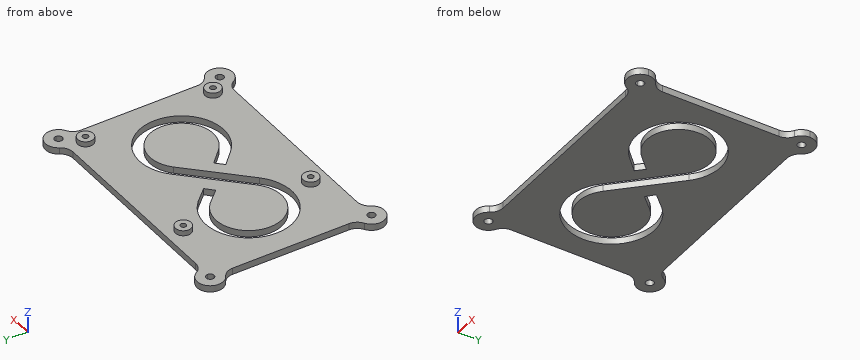
```python
from build123d import *

# Parameters (mm, degrees)
F1_DEPTH = 2.5
F2_R     = 5
F3_R     = 3
F4_DEPTH = 2
F6_D     = 2.2
F6_DEPTH = 3.5
F6_TIP   = 0.6609466809


with BuildPart() as f1:
    # F0 (on Top) → F1 (new body)
    with BuildSketch(Plane.XY):
        with BuildLine():
            ThreePointArc((-45, -26), (-48.5355339059, -34.5355339059), (-40, -31))
            Line((-40, -31), (-43.5, -31))
            ThreePointArc((-43.5, -31), (-46.0606601718, -32.0606601718), (-45, -29.5))
            Line((-45, -29.5), (-45, -26))
        make_face()
        with BuildLine():
            ThreePointArc((-45, -26), (-41.4644660941, -27.4644660941), (-40, -31))
            Line((-40, -31), (40, -31))
            ThreePointArc((40, -31), (41.4644660941, -27.4644660941), (45, -26))
            Line((45, -26), (45, 26))
            ThreePointArc((45, 26), (41.4644660941, 27.4644660941), (40, 31))
            Line((40, 31), (-40, 31))
            ThreePointArc((-40, 31), (-41.4644660941, 27.4644660941), (-45, 26))
            Line((-45, 26), (-45, -26))
        make_face()
        with BuildLine():
            Line((-11.0606601718, -8.9393398282), (8.9393398282, 11.0606601718))
            ThreePointArc((8.9393398282, 11.0606601718), (36.4956890143, -0.3535533906), (8.9393398282, -11.767766953))
            Line((8.9393398282, -11.767766953), (3.7625631329, -6.5909902577))
            Line((3.7625631329, -6.5909902577), (5.1767766953, -5.1767766953))
            Line((5.1767766953, -5.1767766953), (6.5909902577, -3.7625631329))
            Line((6.5909902577, -3.7625631329), (11.767766953, -8.9393398282))
            ThreePointArc((11.767766953, -8.9393398282), (32.4956890143, -0.3535533906), (11.767766953, 8.232233047))
            Line((11.767766953, 8.232233047), (-8.232233047, -11.767766953))
            ThreePointArc((-8.232233047, -11.767766953), (-36.6421356237, 0), (-8.232233047, 11.767766953))
            ThreePointArc((-8.232233047, 11.767766953), (-8.2074655375, 11.7425578811), (-8.1831473235, 11.716915118))
            Line((-8.1831473235, 11.716915118), (-3.3599240188, 6.5401384227))
            Line((-3.3599240188, 6.5401384227), (-4.8232233047, 5.1767766953))
            Line((-4.8232233047, 5.1767766953), (-6.2865225906, 3.8134149679))
            Line((-6.2865225906, 3.8134149679), (-11.0847678218, 8.9633826393))
            ThreePointArc((-11.0847678218, 8.9633826393), (-32.6421241617, -0.0170237742), (-11.0606601718, -8.9393398282))
        make_face(mode=Mode.SUBTRACT)
        with BuildLine():
            Line((-43.5, -31), (-40, -31))
            ThreePointArc((-40, -31), (-41.4644660941, -27.4644660941), (-45, -26))
            Line((-45, -26), (-45, -29.5))
            ThreePointArc((-45, -29.5), (-43.9393398282, -29.9393398282), (-43.5, -31))
        make_face()
        with BuildLine():
            ThreePointArc((45, -26), (41.4644660941, -27.4644660941), (40, -31))
            Line((40, -31), (43.5, -31))
            ThreePointArc((43.5, -31), (43.9393398282, -29.9393398282), (45, -29.5))
            Line((45, -29.5), (45, -26))
        make_face()
        with BuildLine():
            Line((43.5, -31), (40, -31))
            ThreePointArc((40, -31), (45, -36), (50, -31))
            ThreePointArc((50, -31), (48.5355339059, -27.4644660941), (45, -26))
            Line((45, -26), (45, -29.5))
            ThreePointArc((45, -29.5), (46.0606601718, -29.9393398282), (46.5, -31))
            ThreePointArc((46.5, -31), (45, -32.5), (43.5, -31))
        make_face()
        with BuildLine():
            ThreePointArc((-40, 31), (-48.5355339059, 34.5355339059), (-45, 26))
            Line((-45, 26), (-45, 29.5))
            ThreePointArc((-45, 29.5), (-46.0606601718, 32.0606601718), (-43.5, 31))
            Line((-43.5, 31), (-40, 31))
        make_face()
        with BuildLine():
            Line((-45, 29.5), (-45, 26))
            ThreePointArc((-45, 26), (-41.4644660941, 27.4644660941), (-40, 31))
            Line((-40, 31), (-43.5, 31))
            ThreePointArc((-43.5, 31), (-43.9393398282, 29.9393398282), (-45, 29.5))
        make_face()
        with BuildLine():
            ThreePointArc((40, 31), (41.4644660941, 27.4644660941), (45, 26))
            Line((45, 26), (45, 29.5))
            ThreePointArc((45, 29.5), (43.9393398282, 29.9393398282), (43.5, 31))
            Line((43.5, 31), (40, 31))
        make_face()
        with BuildLine():
            Line((45, 29.5), (45, 26))
            ThreePointArc((45, 26), (48.5355339059, 27.4644660941), (50, 31))
            ThreePointArc((50, 31), (45, 36), (40, 31))
            Line((40, 31), (43.5, 31))
            ThreePointArc((43.5, 31), (45, 32.5), (46.5, 31))
            ThreePointArc((46.5, 31), (46.0606601718, 29.9393398282), (45, 29.5))
        make_face()
    extrude(amount=F1_DEPTH)

    # F2
    f2_edges = [f1.edges().sort_by_distance(p)[0] for p in [
        (-40, -31, 1.25),
        (45, 26, 1.25),
        (40, -31, 1.25),
        (-45, -26, 1.25),
        (-45, 26, 1.25),
        (-40, 31, 1.25),
        (40, 31, 1.25),
        (45, -26, 1.25),
    ]]
    fillet(f2_edges, radius=F2_R)

    # F3 (on face) → F4 (join)
    with BuildSketch(Plane.XY.offset(2.5)):
        with Locations((-19, -24.5)):
            Circle(F3_R)
        with Locations((39, -24.5)):
            Circle(F3_R)
        with Locations((39, 24.5)):
            Circle(F3_R)
        with Locations((-19, 24.5)):
            Circle(F3_R)
    extrude(amount=F4_DEPTH)

    # F6
    with Locations(Plane.XY.offset(4.5)):
        with Locations((-19, 24.5), (39, 24.5), (39, -24.5), (-19, -24.5)):
            Hole(F6_D / 2, depth=F6_DEPTH)
            with Locations((0, 0, -(F6_DEPTH + F6_TIP / 2))):  # 118° drill point
                Cone(0, F6_D / 2, F6_TIP, mode=Mode.SUBTRACT)


solid = f1.part
```
Model file for the job. Use its own axes, mm. Give positions to 0.01 mm unless a question says otherwise; leave off trailing zeros. Loops run counter-clockwise (first coordinate to the right, second up) from the corner with the lowest first, then second, coordinate; pieces in that order, holes last. Notation, with made-up numbers: (83.5, 34.25) -> (88.5, 34.25) arc R22 ccw to (88.5, 55.25) -> close; hole circle Ø9 at (-36.5, 57.25). An arc over 180 degrees is marked (long way). Write each question's results on one line, items separated by ' | '.
(1) Probe line 1 along Y through (x, z) = (39, 3.7); line 2 along Y through (x, z) = (-9.5, 1.35); line 3 along Y through (x, z) = (-14, 0.85). List the from-to ranges inside material, lowest first.
Geometry results:
line 1: y = -27.5 to -25.6, -23.4 to -21.5, 21.5 to 23.4, 25.6 to 27.5 | line 2: y = -31 to -12.91, -7.38 to 7.26, 12.91 to 31 | line 3: y = -31 to -15.52, -11.13 to 11.13, 15.52 to 31
(2) Cut at A-A on y = 0. List the corners of the cut face in (x, z).
Geometry results:
outline: (-45, 0) -> (-36.64, 0) -> (-36.64, 2.5) -> (-45, 2.5) -> close; (-32.64, 0) -> (-2.12, 0) -> (-2.12, 2.5) -> (-32.64, 2.5) -> close; (3.54, 0) -> (32.49, 0) -> (32.49, 2.5) -> (3.54, 2.5) -> close; (36.49, 0) -> (45, 0) -> (45, 2.5) -> (36.49, 2.5) -> close
(3) Flat gauge pins, fed straight in: pin 1 Ø1.2 at (y, z) = (7, 1) entering from +X; pin 2 Ø2 at (x, z) = (9, 2) entering from +Y; pin 3 Ø1.5 at (x, z) = (-30.5, 3.5) entering from -Y; pin 4 Ø0.8 at (y, z) = (6, 1.5) entering from -X. Where does each tip first touch, or does it go through?
Geometry results:
pin 1: stops at x = 45 | pin 2: stops at y = 31 | pin 3: passes through | pin 4: stops at x = -45
(4) Cut at B-B on z = 1.8. Give the number of separate pieces and of enclosed holes in the cut face, and give its area (3 significant figures).
Geometry results:
separate pieces: 1 | enclosed holes: 9 | area: 5,070 mm²
